from build123d import *

# Parameters (mm, degrees)
ESBO_O1_W                = 78
ESBO_O1_H                = 74
ESBO_O1_R                = 1.5
ESBO_O1_W_2              = 8
ESBO_O1_H_2              = 24
RESSALTO_EXTRUS_O1_DEPTH = 2.5
CORTE_EXTRUS_O1_DEPTH    = 54.990739947
ESBO_O3_R                = 4
CORTE_EXTRUS_O2_DEPTH    = 10
FILETE1_R                = 5


with BuildPart() as part:
    # Esboço1 → Ressalto-extrusão1 (new, symmetric)
    with BuildSketch(Plane(origin=(0, 0, 0), x_dir=(1, 0, 0), z_dir=(0, 1, 0))):
        Rectangle(ESBO_O1_W, ESBO_O1_H)
        with Locations(Location((-34, 25.5, 0), (0, 0, 270))):
            Circle(ESBO_O1_R, mode=Mode.SUBTRACT)
        with Locations(Location((-16, 25.5, 0), (0, 0, 90))):
            Circle(ESBO_O1_R, mode=Mode.SUBTRACT)
        with Locations(Location((-16, 14.5, 0), (0, 0, 270))):
            Circle(ESBO_O1_R, mode=Mode.SUBTRACT)
        with Locations(Location((-34, 14.5, 0), (0, 0, 90))):
            Circle(ESBO_O1_R, mode=Mode.SUBTRACT)
        with Locations(Location((16, 14.5, 0), (0, 0, 90))):
            Circle(ESBO_O1_R, mode=Mode.SUBTRACT)
        with Locations(Location((16, 25.5, 0), (0, 0, 270))):
            Circle(ESBO_O1_R, mode=Mode.SUBTRACT)
        with Locations(Location((34, 14.5, 0), (0, 0, 270))):
            Circle(ESBO_O1_R, mode=Mode.SUBTRACT)
        with Locations(Location((34, 25.5, 0), (0, 0, 90))):
            Circle(ESBO_O1_R, mode=Mode.SUBTRACT)
        with Locations(Location((34, -14.5, 0), (0, 0, 90))):
            Circle(ESBO_O1_R, mode=Mode.SUBTRACT)
        with Locations(Location((16, -14.5, 0), (0, 0, 270))):
            Circle(ESBO_O1_R, mode=Mode.SUBTRACT)
        with Locations(Location((34, -25.5, 0), (0, 0, 270))):
            Circle(ESBO_O1_R, mode=Mode.SUBTRACT)
        with Locations(Location((16, -25.5, 0), (0, 0, 90))):
            Circle(ESBO_O1_R, mode=Mode.SUBTRACT)
        with Locations(Location((-16, -14.5, 0), (0, 0, 90))):
            Circle(ESBO_O1_R, mode=Mode.SUBTRACT)
        with Locations(Location((-16, -25.5, 0), (0, 0, 270))):
            Circle(ESBO_O1_R, mode=Mode.SUBTRACT)
        with Locations(Location((-34, -14.5, 0), (0, 0, 270))):
            Circle(ESBO_O1_R, mode=Mode.SUBTRACT)
        with Locations(Location((-34, -25.5, 0), (0, 0, 90))):
            Circle(ESBO_O1_R, mode=Mode.SUBTRACT)
        with Locations((-25, 20)):
            Rectangle(ESBO_O1_W_2, ESBO_O1_H_2, mode=Mode.SUBTRACT)
        with Locations((25, 20)):
            Rectangle(ESBO_O1_W_2, ESBO_O1_H_2, mode=Mode.SUBTRACT)
        with Locations((25, -20)):
            Rectangle(ESBO_O1_W_2, ESBO_O1_H_2, mode=Mode.SUBTRACT)
        with Locations((-25, -20)):
            Rectangle(ESBO_O1_W_2, ESBO_O1_H_2, mode=Mode.SUBTRACT)
    extrude(amount=RESSALTO_EXTRUS_O1_DEPTH, both=True)

    # Esboço2 → Corte-extrusão1 (cut, symmetric)
    with BuildSketch(Plane(origin=(0, 2.5, 0), x_dir=(1, 0, 0), z_dir=(0, 1, 0))):
        Polygon((-4.584870607, -13.571957621), (-21.450620651, -37), (21.450620651, -37), (4.584870607, -13.571957621), align=None)
    corte_extrus_o1 = extrude(amount=CORTE_EXTRUS_O1_DEPTH, both=True, mode=Mode.SUBTRACT)

    # Espelhar1: Corte-extrusão1 across plane
    add(corte_extrus_o1.mirror(Plane.XY), mode=Mode.SUBTRACT)

    # Esboço3 → Corte-extrusão2 (cut)
    with BuildSketch(Plane(origin=(0, 2.5, 0), x_dir=(1, 0, 0), z_dir=(0, 1, 0))):
        with Locations(Location((-4, 0, 0), (0, 0, 270))):
            Circle(ESBO_O3_R)
        with BuildLine():
            Line((-32, 3), (-15, 3))
            ThreePointArc((-15, 3), (-12, 0), (-15, -3))
            Line((-15, -3), (-32, -3))
            ThreePointArc((-32, -3), (-35, 0), (-32, 3))
        make_face()
        with BuildLine():
            Line((32, 3), (15, 3))
            ThreePointArc((15, 3), (12, 0), (15, -3))
            Line((15, -3), (32, -3))
            ThreePointArc((32, -3), (35, 0), (32, 3))
        make_face()
    extrude(amount=-CORTE_EXTRUS_O2_DEPTH, mode=Mode.SUBTRACT)

    # Filete1
    filete1_edges = [part.edges().sort_by_distance(p)[0] for p in [
        (21.450620651, 0, 37),
        (-21.450620651, 0, 37),
        (-4.584870607, 0, 13.571957621),
        (4.584870607, 0, 13.571957621),
        (21.450620651, 0, -37),
        (-21.450620651, 0, -37),
        (4.584870607, 0, -13.571957621),
        (-4.584870607, 0, -13.571957621),
        (39, 0, 37),
        (-39, 0, 37),
        (-39, 0, -37),
        (39, 0, -37),
    ]]
    fillet(filete1_edges, radius=FILETE1_R)


solid = part.part
Geometry: final body of the model. Coordinates: model frame, mm. A direction names the side the tool comes from. Coordinates: 2 decimals unless noted, no trailing zeros. Order: outer loops, then holes, each group sorted by start corner. A loop starts at its lowest first (then second) coordinate and runs counter-clockwise, first axis right, second up.
(1) Draft query along Z for faces 1 (the face through (-12.92, 0.04, -25.15)), 2 (the face through (-9, 2.5, -1)), 3 (the face through (21, 0, -20)). Return one class per face: pulls with the +Z half, pulls with the -Z half, needs draft (parallel to the pull), parting line crosses it, or undercut.
(2) Section query B-B (x = -16). Return the cut outline in (y, z), plus the area to 3 significant figures.
(3) First-contact query: pin 1 (1.8 mm diameter, centred on x = 16, z = 25.5, fed in from -Y). Flat tip, straight axial feed; report the tip coordinate or a pass-through.
(4) Section query A-A (z = 0). Return the cut outline in (x, y), plus the area to 3 significant figures.
(5) Section query C-C (z = 10). Return the cut outline in (x, y), plus the area to 3 significant figures.
(6) Material intervals for probe 1 along X at (y, z) = (0.85, -12); probe 2 along X at (y, z) = (0.8, 0); probe 3 along Z at (x, y) = (15.5, -1), sorted ascending.
(7) Section query D-D (x = -4). Return the cut outline in (y, z).
(8) Access query for faces 4 (the face through (13.1, 0, -25.4)), 5 (the face through (-21.762, 0.035, 36.465)), 6 (the face through (35, 0, 0)). Directions: +Z, -Z, +X, -X, +Y, -Y. A direction counts if a zero-diameter tool reaches every point of the face in a straight line with its end or side. Return the directions, or none.
Solution:
1. face 1: pulls with the -Z half
1. face 2: needs draft
1. face 3: undercut
2. outline: (-2.5, -29.43) - (2.5, -29.43) - (2.5, -27) - (-2.5, -27) - close; (-2.5, -24) - (2.5, -24) - (2.5, -16) - (-2.5, -16) - close; (-2.5, -13) - (2.5, -13) - (2.5, -3) - (-2.5, -3) - close; (-2.5, 3) - (2.5, 3) - (2.5, 13) - (-2.5, 13) - close; (-2.5, 16) - (2.5, 16) - (2.5, 24) - (-2.5, 24) - close; (-2.5, 27) - (2.5, 27) - (2.5, 29.43) - (-2.5, 29.43) - close
2. area: 204 mm2
3. pin 1: passes through
4. outline: (-39, -2.5) - (-35, -2.5) - (-35, 2.5) - (-39, 2.5) - close; (-12, -2.5) - (-8, -2.5) - (-8, 2.5) - (-12, 2.5) - close; (0, -2.5) - (12, -2.5) - (12, 2.5) - (0, 2.5) - close; (35, -2.5) - (39, -2.5) - (39, 2.5) - (35, 2.5) - close
4. area: 120 mm2
5. outline: (-39, -2.5) - (-29, -2.5) - (-29, 2.5) - (-39, 2.5) - close; (-21, -2.5) - (21, -2.5) - (21, 2.5) - (-21, 2.5) - close; (29, -2.5) - (39, -2.5) - (39, 2.5) - (29, 2.5) - close
5. area: 310 mm2
6. probe 1: x = -39 to -29, -21 to 21, 29 to 39
6. probe 2: x = -39 to -35, -12 to -8, 0 to 12, 35 to 39
6. probe 3: z = -28.73 to -26.91, -24.09 to -15.91, -13.09 to -3, 3 to 13.09, 15.91 to 24.09, 26.91 to 28.73
7. outline: (-2.5, -13.98) - (2.5, -13.98) - (2.5, -4) - (-2.5, -4) - close; (-2.5, 4) - (2.5, 4) - (2.5, 13.98) - (-2.5, 13.98) - close
8. face 4: -Z, +Y, -Y
8. face 5: +Z, +Y, -Y
8. face 6: +Y, -Y
